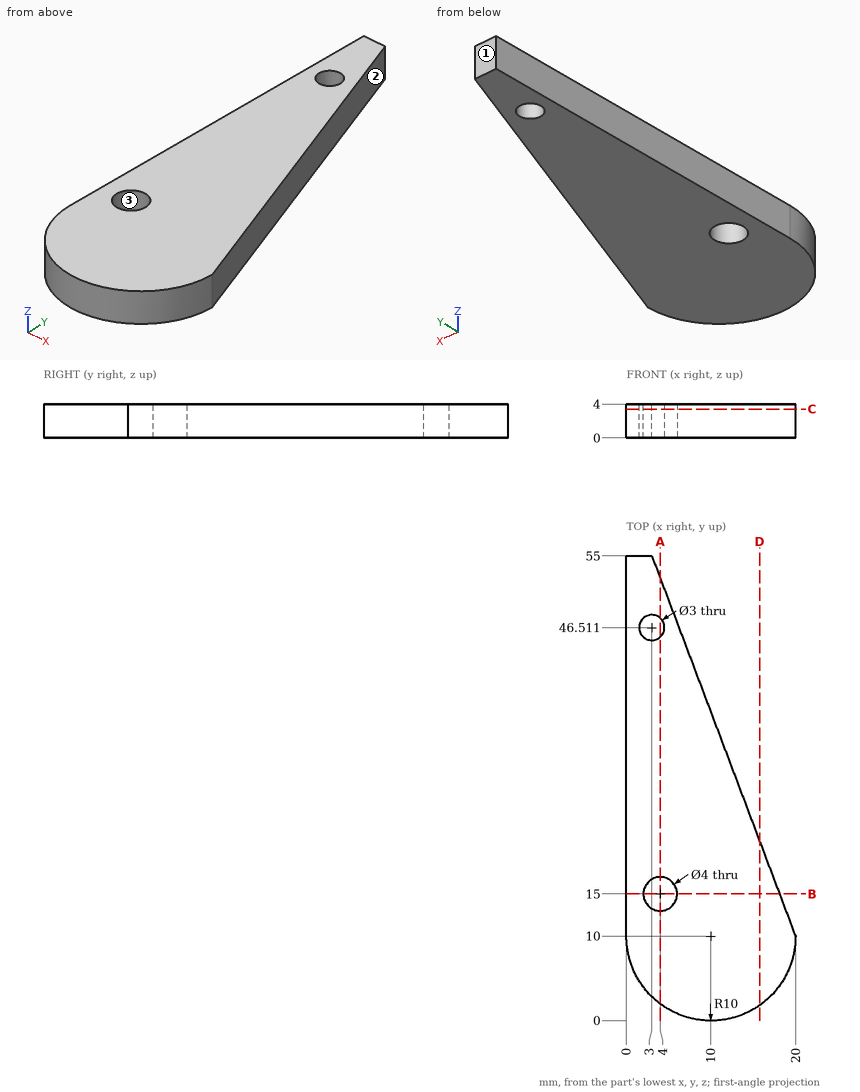
Part print with two shaded views. Sizes in mm from the minimum x, y, z corner. Give positions to 0.01 mm unless a question says otherwise; leave off trailing zeros. Write each loop counter-clockwise with the first axis right and the second up, starting at its lowest first coordinate (ties: lowest second). Pieces come first, ordered by that corner, then holes.
1) Probe L1, parallel to X at y = 51, z = 2.6; L2, parallel to X at y = 14, z = 3.45; L3, parallel to Y at x = 1.75, z = 0.85. List the from-to ranges inside material, lowest first.
Resolved:
L1: x = 0 to 4.51
L2: x = 0 to 2.27, 5.73 to 18.49
L3: y = 4.35 to 45.68, 47.34 to 55
2) Two-plate mould, pull along X, no slides. Class the marked faces 1, 2 and 3: released by +X, released by -X, zero draft, split by the parting line, or undercut.
Resolved:
face 1: zero draft
face 2: released by +X
face 3: undercut
3) Cut at A-A on x = 4. Write the cut outline in (y, z), then the cut area to 3 significant figures.
Resolved:
outline: (2, 0) - (13, 0) - (13, 4) - (2, 4) - close; (17, 0) - (45.39, 0) - (45.39, 4) - (17, 4) - close; (47.63, 0) - (52.35, 0) - (52.35, 4) - (47.63, 4) - close
area: 176 mm2
4) Cut at C-C on z = 3.4. Write the cut outline in (x, y), then the cut area to 3 significant figures.
Resolved:
outline: (0, 10) arc R10 ccw to (20, 10) - (3, 55) - (0, 55) - close; hole circle Ø3 at (3, 46.51); hole circle Ø4 at (4, 15)
area: 655 mm2
5) Pin check, flat tips, straight feed: pin 1 (3 mm diameter, centred on x = 4, y = 15, fed in from -Z); pin 2 (1.5 mm diameter, centred on x = 3.5, z = 2, fed in from -Y); pin 3 (1.5 mm diameter, centred on y = 21.5, z = 2.5, fed in from +X). Stop position of each tip, or through.
Resolved:
pin 1: passes through
pin 2: stops at y = 1.82
pin 3: stops at x = 15.94
6) Cut at B-B on y = 15. Write the cut outline in (x, z).
Resolved:
outline: (0, 0) - (2, 0) - (2, 4) - (0, 4) - close; (6, 0) - (18.11, 0) - (18.11, 4) - (6, 4) - close
7) Cut at D-D on x = 15.75. Write the cut outline in (y, z).
Resolved:
outline: (1.82, 0) - (21.25, 0) - (21.25, 4) - (1.82, 4) - close
